from build123d import *

# Parameters (mm, degrees)
BOSS_EXTRUDE1_DEPTH = 10
FILLET1_R           = 2
FILLET2_R           = 2
SKETCH2_W           = 150.559508978
SKETCH2_H           = 227.088218296
CUT_EXTRUDE1_DEPTH  = 1
BOSS_EXTRUDE2_DEPTH = 20
SKETCH4_W           = 6.725754883
SKETCH4_H           = 15
CUT_EXTRUDE2_DEPTH  = 5
SKETCH5_W           = 10.823402452
SKETCH5_H           = 30.328045867
SKETCH5_W_2         = 7.884028191
SKETCH5_H_2         = 2.324389301
CUT_EXTRUDE3_DEPTH  = 5
SKETCH6_R           = 4.682007924
BOSS_EXTRUDE3_DEPTH = 2
CUT_EXTRUDE4_DEPTH  = 1
SKETCH8_R           = 3.203249508
BOSS_EXTRUDE4_DEPTH = 5
SKETCH9_R           = 2.554506396
SKETCH9_R_2         = 0.710039237
CUT_EXTRUDE5_DEPTH  = 5
SKETCH10_R          = 3.699360335
CUT_EXTRUDE6_DEPTH  = 5
BOSS_EXTRUDE5_DEPTH = 2
SKETCH12_R          = 3.630842339
BOSS_EXTRUDE6_DEPTH = 4
SKETCH13_R          = 1
CUT_EXTRUDE7_DEPTH  = 2


with BuildPart() as part:
    # Sketch1 → Boss-Extrude1 (new body)
    with BuildSketch(Plane.XY):
        with BuildLine():
            Line((-10.72344857, 42.703899352), (146.86655143, 42.703899352))
            ThreePointArc((146.86655143, 42.703899352), (156.04479745, 38.902145372), (159.84655143, 29.723899352))
            Line((159.84655143, 29.723899352), (159.84655143, -210.266100648))
            ThreePointArc((159.84655143, -210.266100648), (156.04479745, -219.444346668), (146.86655143, -223.246100648))
            Line((146.86655143, -223.246100648), (-10.72344857, -223.246100648))
            ThreePointArc((-10.72344857, -223.246100648), (-19.90169459, -219.444346668), (-23.70344857, -210.266100648))
            Line((-23.70344857, -210.266100648), (-23.70344857, 29.723899352))
            ThreePointArc((-23.70344857, 29.723899352), (-19.90169459, 38.902145372), (-10.72344857, 42.703899352))
        make_face()
    extrude(amount=BOSS_EXTRUDE1_DEPTH)

    # Fillet1
    fillet1_edges = [part.edges().sort_by_distance(p)[0] for p in [
        (156.04479745, -219.444346668, 10),
        (159.84655143, -90.271100648, 10),
        (156.04479745, 38.902145372, 10),
        (68.07155143, 42.703899352, 10),
        (-19.90169459, 38.902145372, 10),
        (-23.70344857, -90.271100648, 10),
        (-19.90169459, -219.444346668, 10),
        (68.07155143, -223.246100648, 10),
    ]]
    fillet(fillet1_edges, radius=FILLET1_R)

    # Fillet2
    fillet2_edges = [part.edges().sort_by_distance(p)[0] for p in [
        (68.07155143, -223.246100648, 0),
        (-19.90169459, -219.444346668, 0),
        (-23.70344857, -90.271100648, 0),
        (-19.90169459, 38.902145372, 0),
        (68.07155143, 42.703899352, 0),
        (156.04479745, 38.902145372, 0),
        (159.84655143, -90.271100648, 0),
        (156.04479745, -219.444346668, 0),
    ]]
    fillet(fillet2_edges, radius=FILLET2_R)

    # Sketch2 → Cut-Extrude1 (cut)
    with BuildSketch(Plane.XY.offset(10)):
        with Locations((68.657611098, -91.510541064)):
            Rectangle(SKETCH2_W, SKETCH2_H)
    extrude(amount=-CUT_EXTRUDE1_DEPTH, mode=Mode.SUBTRACT)

    # Sketch3 → Boss-Extrude2 (add)
    with BuildSketch(Plane(origin=(0, 0, 0), x_dir=(-1, 0, 0), z_dir=(0, 0, -1))):
        with BuildLine():
            Line((-102.58655143, -13.276100648), (-33.54655143, -13.276100648))
            ThreePointArc((-33.54655143, -13.276100648), (-24.36830541, -17.077854628), (-20.56655143, -26.256100648))
            Line((-20.56655143, -26.256100648), (-20.56655143, -158.296100648))
            ThreePointArc((-20.56655143, -158.296100648), (-24.36830541, -167.474346668), (-33.54655143, -171.276100648))
            Line((-33.54655143, -171.276100648), (-102.58655143, -171.276100648))
            ThreePointArc((-102.58655143, -171.276100648), (-111.76479745, -167.474346668), (-115.56655143, -158.296100648))
            Line((-115.56655143, -158.296100648), (-115.56655143, -26.256100648))
            ThreePointArc((-115.56655143, -26.256100648), (-111.76479745, -17.077854628), (-102.58655143, -13.276100648))
        make_face()
    extrude(amount=BOSS_EXTRUDE2_DEPTH)

    # Sketch4 → Cut-Extrude2 (cut)
    with BuildSketch(Plane(origin=(115.56655143, 0, 0), x_dir=(0, 0, -1), z_dir=(1, 0, 0))):
        with Locations((10.383044541, -78.756100648)):
            Rectangle(SKETCH4_W, SKETCH4_H)
        with Locations((10.383044541, -98.756100648)):
            Rectangle(SKETCH4_W, SKETCH4_H)
        with Locations((10.383044541, -118.756100648)):
            Rectangle(SKETCH4_W, SKETCH4_H)
        with Locations((10.383044541, -138.756100648)):
            Rectangle(SKETCH4_W, SKETCH4_H)
    extrude(amount=-CUT_EXTRUDE2_DEPTH, mode=Mode.SUBTRACT)

    # Sketch5 → Cut-Extrude3 (cut)
    with BuildSketch(Plane(origin=(115.56655143, 0, 0), x_dir=(0, 0, -1), z_dir=(1, 0, 0))):
        with Locations((8.435417198, -48.817241241)):
            Rectangle(SKETCH5_W, SKETCH5_H)
        with Locations((8.473269779, -40.058791114)):
            Rectangle(SKETCH5_W_2, SKETCH5_H_2, mode=Mode.SUBTRACT)
        with Locations((8.473269779, -37.058791114)):
            Rectangle(SKETCH5_W_2, SKETCH5_H_2, mode=Mode.SUBTRACT)
        with Locations((8.473269779, -43.058791114)):
            Rectangle(SKETCH5_W_2, SKETCH5_H_2, mode=Mode.SUBTRACT)
        with Locations((8.473269779, -46.058791114)):
            Rectangle(SKETCH5_W_2, SKETCH5_H_2, mode=Mode.SUBTRACT)
        with Locations((8.473269779, -49.058791114)):
            Rectangle(SKETCH5_W_2, SKETCH5_H_2, mode=Mode.SUBTRACT)
        with Locations((8.473269779, -52.058791114)):
            Rectangle(SKETCH5_W_2, SKETCH5_H_2, mode=Mode.SUBTRACT)
        with Locations((8.473269779, -55.058791114)):
            Rectangle(SKETCH5_W_2, SKETCH5_H_2, mode=Mode.SUBTRACT)
        with Locations((8.473269779, -58.058791114)):
            Rectangle(SKETCH5_W_2, SKETCH5_H_2, mode=Mode.SUBTRACT)
        with Locations((8.473269779, -61.058791114)):
            Rectangle(SKETCH5_W_2, SKETCH5_H_2, mode=Mode.SUBTRACT)
    extrude(amount=-CUT_EXTRUDE3_DEPTH, mode=Mode.SUBTRACT)

    # Sketch6 → Boss-Extrude3 (add)
    with BuildSketch(Plane(origin=(115.56655143, 0, 0), x_dir=(0, 0, -1), z_dir=(1, 0, 0))):
        with Locations((9.515417979, -152.907768045)):
            Circle(SKETCH6_R)
    extrude(amount=BOSS_EXTRUDE3_DEPTH)

    # Sketch7 → Cut-Extrude4 (cut)
    with BuildSketch(Plane(origin=(117.56655143, 0, 0), x_dir=(0, 0, -1), z_dir=(1, 0, 0))):
        with BuildLine():
            ThreePointArc((11.805414658, -154.310979404), (6.626563337, -152.860959544), (11.818169697, -151.457292202))
            Line((11.818169697, -151.457292202), (12.404150804, -151.228337022))
            ThreePointArc((12.404150804, -151.228337022), (6.003985158, -152.87342514), (12.404150804, -154.518513257))
            Line((12.404150804, -154.518513257), (11.805414658, -154.310979404))
        make_face()
        with BuildLine():
            Line((12.18490875, -152.543842862), (9.037284105, -152.543842862))
            Line((9.037284105, -152.543842862), (9.037284105, -153.351490318))
            Line((9.037284105, -153.351490318), (12.163172337, -153.351490318))
            ThreePointArc((12.163172337, -153.351490318), (12.194112354, -153.113347139), (12.204451244, -152.87342514))
            ThreePointArc((12.204451244, -152.87342514), (12.199561333, -152.708344563), (12.18490875, -152.543842862))
        make_face()
        with BuildLine():
            Line((12.811043942, -152.543842862), (12.18490875, -152.543842862))
            ThreePointArc((12.18490875, -152.543842862), (12.199561333, -152.708344563), (12.204451244, -152.87342514))
            ThreePointArc((12.204451244, -152.87342514), (12.194112354, -153.113347139), (12.163172337, -153.351490318))
            Line((12.163172337, -153.351490318), (12.793339111, -153.351490318))
            ThreePointArc((12.793339111, -153.351490318), (12.818575546, -153.113049573), (12.827001565, -152.87342514))
            ThreePointArc((12.827001565, -152.87342514), (12.823009824, -152.708440956), (12.811043942, -152.543842862))
        make_face()
        with BuildLine():
            Line((13.705368282, -152.543842862), (12.811043942, -152.543842862))
            ThreePointArc((12.811043942, -152.543842862), (12.823009824, -152.708440956), (12.827001565, -152.87342514))
            ThreePointArc((12.827001565, -152.87342514), (12.818575546, -153.113049573), (12.793339111, -153.351490318))
            Line((12.793339111, -153.351490318), (13.705368282, -153.351490318))
            Line((13.705368282, -153.351490318), (13.705368282, -152.543842862))
        make_face()
    extrude(amount=-CUT_EXTRUDE4_DEPTH, mode=Mode.SUBTRACT)

    # Sketch8 → Boss-Extrude4 (add)
    with BuildSketch(Plane.XZ.offset(171.276100648)):
        with Locations((39.948285329, -5.670763906)):
            Circle(SKETCH8_R)
    extrude(amount=BOSS_EXTRUDE4_DEPTH)

    # Sketch9 → Cut-Extrude5 (cut)
    with BuildSketch(Plane.XZ.offset(176.276100648)):
        with Locations((39.948285329, -5.670763906)):
            Circle(SKETCH9_R)
        with Locations((39.948285329, -5.670763906)):
            Circle(SKETCH9_R_2, mode=Mode.SUBTRACT)
    extrude(amount=-CUT_EXTRUDE5_DEPTH, mode=Mode.SUBTRACT)

    # Sketch10 → Cut-Extrude6 (cut)
    with BuildSketch(Plane.XZ.offset(171.276100648)):
        with Locations((49.940704465, -5.30990755)):
            Circle(SKETCH10_R)
    extrude(amount=-CUT_EXTRUDE6_DEPTH, mode=Mode.SUBTRACT)

    # Sketch11 → Boss-Extrude5 (add)
    with BuildSketch(Plane.ZY.offset(-20.56655143)):
        Polygon((-6.82408612, -143.759373329), (-11.294019493, -146.340090565), (-11.294019493, -151.501525037), (-6.82408612, -154.082242272), (-2.354152748, -151.501525037), (-2.354152748, -146.340090565), align=None)
    extrude(amount=BOSS_EXTRUDE5_DEPTH)

    # Sketch12 → Boss-Extrude6 (add)
    with BuildSketch(Plane.ZY.offset(-18.56655143)):
        with Locations((-6.577483045, -148.906392161)):
            Circle(SKETCH12_R)
    extrude(amount=BOSS_EXTRUDE6_DEPTH)

    # Sketch13 → Cut-Extrude7 (cut)
    with BuildSketch(Plane(origin=(0, 0, 0), x_dir=(-1, 0, 0), z_dir=(0, 0, -1))):
        with Locations((-105.84655143, -185.246100648)):
            Circle(SKETCH13_R)
        with Locations((-30.84655143, -185.246100648)):
            Circle(SKETCH13_R)
    extrude(amount=-CUT_EXTRUDE7_DEPTH, mode=Mode.SUBTRACT)


solid = part.part
Work out the finished part from the listing and answer in its coordinate system (mm). A direction names the side the tool comes from. Coordinates: 2 decimals unless noted, no trailing zeros. Write each loop counter-clockwise with the first axis right and the second up, starting at its lowest first coordinate (ties: lowest second). Pieces come first, ordered by that corner, then holes. Notation, with made-up numbers: (18.5, 41) - (42.5, 41) arc R14 cw to (42.5, 66) - close; hole circle Ø3 at (47.5, 42.25). An arc over 180 degrees is marked (long way). One line per question, with ' | ' between items.
1) The mould has two halves that part along Y. Classify faces 5 (the face through (-20, 38.8, 5)), 6 (the face through (116.553, -148.266, -8.906)), 7 (the face through (117.074, -152.963, -6.628)): +Y half, -Y half, draft (parallel to the pull), parting line (faces both ways), or undercut.
Checks:
face 5: +Y half | face 6: parting line | face 7: undercut
2) Consider probe 1 along Z at (x, y) = (-14, -41); probe 2 along X at (y, z) = (-149, -15); probe 3 along Z at (x, y) = (4, -175). Determine where each line is inside the solid, lowest interval first. Write a range as [from, to].
Checks:
probe 1: [0, 10] | probe 2: [20.57, 115.57] | probe 3: [0, 9]
3) Flat-ended cylindrical pins translate along their axes: P1, Ø6, axis at y = -116.5, z = -13, coming from the +X side; P2, Ø0.7, axis at x = 113.5, y = -48.5, coming from the +Z side; P3, Ø1.5, axis at x = 112, z = -10, coming from the -Y side. Find the tip coordinate at first contact, or state that the pin passes through.
Checks:
P1: x = 115.57 | P2: z = 9 | P3: y = -167.96
4) Find section B-B, the plane x = 137. Determine the outline of the cut face in (y, z).
Checks:
outline: (-223.25, 2) arc R2 ccw to (-221.25, 0) - (40.7, 0) arc R2 ccw to (42.7, 2) - (42.7, 8) arc R2 ccw to (40.7, 10) - (22.03, 10) - (22.03, 9) - (-205.05, 9) - (-205.05, 10) - (-221.25, 10) arc R2 ccw to (-223.25, 8) - close
5) Find section C-C, the plane x = 71. Determine the outline of the cut face in (y, z), and give its area (3 significant figures).
Checks:
outline: (-223.25, 2) arc R2 ccw to (-221.25, 0) - (-171.28, 0) - (-171.28, -20) - (-13.28, -20) - (-13.28, 0) - (40.7, 0) arc R2 ccw to (42.7, 2) - (42.7, 8) arc R2 ccw to (40.7, 10) - (22.03, 10) - (22.03, 9) - (-205.05, 9) - (-205.05, 10) - (-221.25, 10) arc R2 ccw to (-223.25, 8) - close | area: 5,590 mm2
6) For faces 1 (the face through (111.865, -17.179, -9.86)), 2 (the face through (16.59, -152.45, -7.36)), 3 (the face through (42.907, -173.741, -6.898)), 4 (the face through (113, -91.256, -10)), determine the directions among +Z, -Z, +X, -X, +Y, -Y from which every point of the face is accessible in a straight line to the end or side of a thin tool.
Checks:
face 1: -Z, +X, +Y | face 2: -X | face 3: -Y | face 4: +X
7) Find section A-A, the plane y = -137. Determine the outline of the cut face in (x, z).
Checks:
outline: (-23.7, 2) arc R2 ccw to (-21.7, 0) - (20.57, 0) - (20.57, -20) - (115.57, -20) - (115.57, -13.75) - (110.57, -13.75) - (110.57, -7.02) - (115.57, -7.02) - (115.57, 0) - (157.85, 0) arc R2 ccw to (159.85, 2) - (159.85, 8) arc R2 ccw to (157.85, 10) - (143.94, 10) - (143.94, 9) - (-6.62, 9) - (-6.62, 10) - (-21.7, 10) arc R2 ccw to (-23.7, 8) - close
